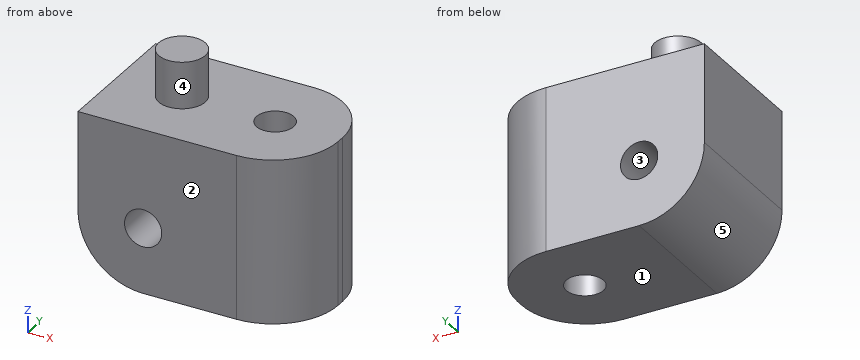
```python
from build123d import *

# Parameters (mm, degrees)
F0_W     = 12
F0_H     = 7.4
F1_DEPTH = 8.8
F2_R     = 1
F3_DEPTH = 25
F4_R     = 3.5
F5_R     = 3.5
F6_R     = 1.25
F7_DEPTH = 2.5
F6_R_2   = 1
F8_DEPTH = 25


with BuildPart() as f1:
    # F0 (on Top) → F1 (new body)
    with BuildSketch(Plane.XY):
        with Locations((6, 3.7)):
            Rectangle(F0_W, F0_H)
    extrude(amount=F1_DEPTH)

    # F2 (on face) → F3 (cut)
    with BuildSketch(Plane.XZ):
        with Locations((3.5, 3.5)):
            Circle(F2_R)
    extrude(amount=-F3_DEPTH, mode=Mode.SUBTRACT)

    # F4
    f4_edges = [f1.edges().sort_by_distance(p)[0] for p in [
        (0, 3.7, 0),
    ]]
    fillet(f4_edges, radius=F4_R)

    # F5
    f5_edges = [f1.edges().sort_by_distance(p)[0] for p in [
        (12, 0, 4.4),
        (12, 7.4, 4.4),
    ]]
    fillet(f5_edges, radius=F5_R)

    # F6 (on face) → F7 (join)
    with BuildSketch(Plane.XY.offset(8.8)):
        with Locations((3.5, 3.7)):
            Circle(F6_R)
    extrude(amount=F7_DEPTH)

    # F6 (on face) → F8 (cut)
    with BuildSketch(Plane.XY.offset(8.8)):
        with Locations((8.5, 3.7)):
            Circle(F6_R_2)
    extrude(amount=-F8_DEPTH, mode=Mode.SUBTRACT)


solid = f1.part
```
Verification items for the finished model (mm, model axes). Face numbers are marked on the shaded views. A direction names the side the tool comes from. Round coordinates to 2 decimals unless told otherwise and drop trailing zeros. Order: outer loops, then holes, each group sorted by start corner. A loop starts at its lowest first (then second) coordinate and runs counter-clockwise, first axis right, second up. Notation, with made-up numbers: (-14, -1) -> (6, -1) arc R17 cw to (6, 26) -> close; hole circle Ø3 at (-28.75, -34.5). An arc over 180 degrees is marked (long way). Put each result on its own line as item: value. Start each with the question number.
(1) Section check B-B (z = 6). Enter the section's corners in (x, y).
(2) Section check C-C (z = 3.75). Enter the section's corners in (x, y), then the cut area to 3 significant figures.
(3) Draft check along Z on the marked faces 1, 2 and 3. Enter one of: +Z half, -Z half, draft (parallel to the pull), parting line (faces both ways), or undercut.
(4) Depth check by flat-ended pin: pin 1 Ø1.2 at (x, y) = (8.5, 3.7) entering from -Z; pin 2 Ø2 at (y, z) = (5.5, 3.5) entering from +X. Enter the tip coordinate at first touch or a pass-through.
(5) Section check A-A (y = 3.7). Enter the section's corners in (x, z), then the cut area to 3 significant figures.
(6) Section check D-D (x = 4). Enter the section's corners in (y, z).
(7) Material ranges on line 1 along Y through (x, z) = (8.5, 4.5); line 2 along Z through (x, y) = (3.5, 4.5); line 3 along Z through (x, y) = (3.5, 5.5), recorded low to high.
(8) Tool access check on the marked faces 4 and 5. Record the directions out of +Z, -Z, +X, -X, +Y, -Y that give a thin tool (end or side, any length) a straight path to the whole face; none if there is none.
Completed:
1. outline: (0, 0) -> (8.5, 0) arc R3.5 ccw to (12, 3.5) -> (12, 3.9) arc R3.5 ccw to (8.5, 7.4) -> (0, 7.4) -> close; hole circle Ø2 at (8.5, 3.7)
2. outline: (0, 0) -> (2.53, 0) -> (2.53, 7.4) -> (0, 7.4) -> close; (4.47, 0) -> (8.5, 0) arc R3.5 ccw to (12, 3.5) -> (12, 3.9) arc R3.5 ccw to (8.5, 7.4) -> (4.47, 7.4) -> close; hole circle Ø2 at (8.5, 3.7)
2. area: 66.1 mm2
3. face 1: -Z half
3. face 2: draft
3. face 3: undercut
4. pin 1: passes through
4. pin 2: stops at x = 11.95
5. outline: (0, 3.5) arc R3.5 ccw to (3.5, 0) -> (7.5, 0) -> (7.5, 8.8) -> (4.75, 8.8) -> (4.75, 11.3) -> (2.25, 11.3) -> (2.25, 8.8) -> (0, 8.8) -> close; (9.5, 0) -> (12, 0) -> (12, 8.8) -> (9.5, 8.8) -> close; hole circle Ø2 at (3.5, 3.5)
5. area: 88.5 mm2
6. outline: (0, 0) -> (7.4, 0) -> (7.4, 2.63) -> (0, 2.63) -> close; (0, 4.37) -> (7.4, 4.37) -> (7.4, 8.8) -> (4.85, 8.8) -> (4.85, 11.3) -> (2.55, 11.3) -> (2.55, 8.8) -> (0, 8.8) -> close
7. line 1: y = 0 to 2.7, 4.7 to 7.4
7. line 2: z = 0 to 2.5, 4.5 to 11.3
7. line 3: z = 0 to 2.5, 4.5 to 8.8
8. face 4: +Z
8. face 5: -Z, -X, +Y, -Y
